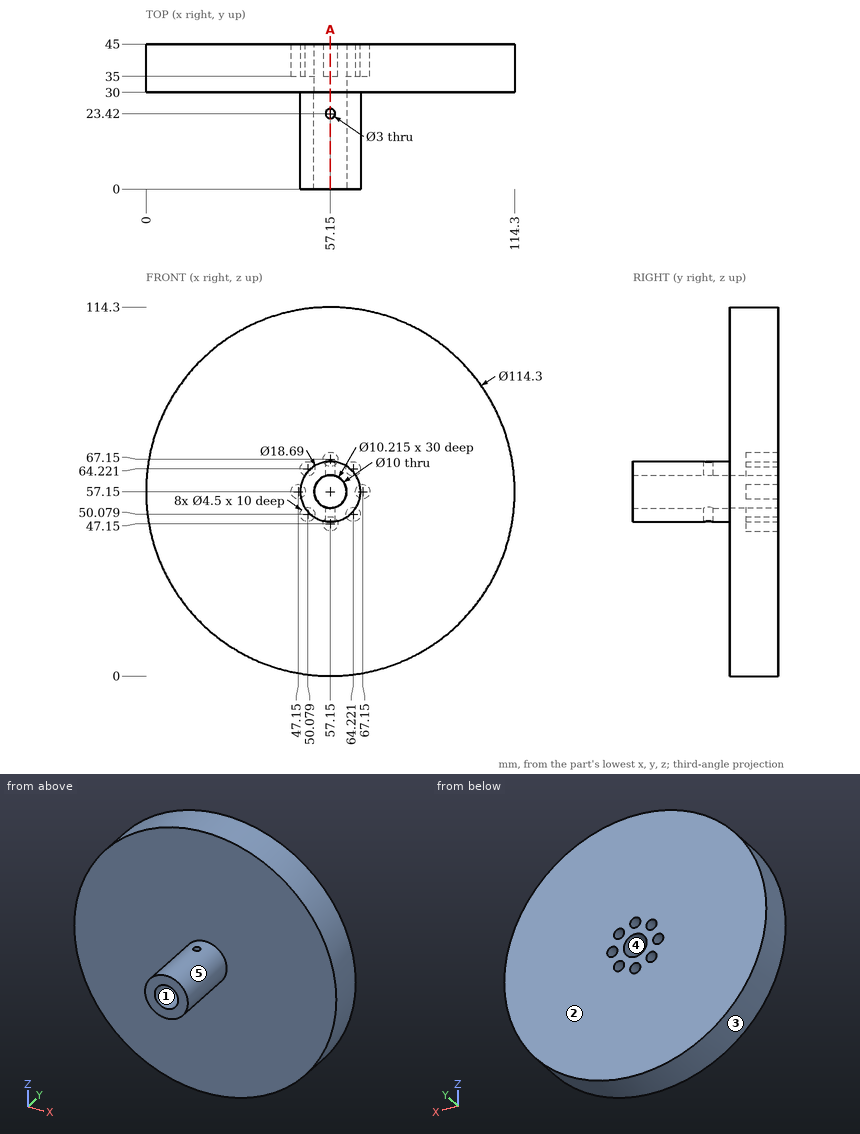
Verification items for this drawing (mm, ordinates from the low corner). A direction names the side the tool comes from. Round coordinates to 2 decimals unless told otherwise and drop trailing zeros. Use one line per item in the form item = value.
1. Go/stop test with flat-tipped pins: pin 1 (2 mm diameter, centred on x = 50.5, z = 51, fed in from +Y); pin 2 (6 mm diameter, centred on x = 84.5, y = 28.5, fed in from -Z); pin 3 (3 mm diameter, centred on y = 39, z = 81, fed in from -X); pin 4 (1.8 mm diameter, centred on x = 57.15, y = 23.42, fed in from +Z). Record where each tip stops, or that it passes through.
Working result:
pin_1 = 35
pin_2 = 5.64
pin_3 = 4.55
pin_4 = through
2. Cross-section at A-A, the plane x = 57.15. Count the separate pieces of the cut face and the enclosed holes in it, plus the area to 3 significant figures.
Working result:
separate_pieces = 4
enclosed_holes = 0
area = 1,700 mm^2
3. Mould release check, pull along X, two halves, no side actions. Record for the marked faces 1, 2 and 3: pulls with the +X half, pulls with the -X half, needs draft (parallel to the pull), parting line crosses it, or undercut.
Working result:
face_1 = undercut
face_2 = needs draft
face_3 = parting line crosses it
4. Set-up check for the marked faces 4 and 5: record each of +Z, -Z, +X, -X, +Y, -Y from which the full face is reachable in a straight line by a thin tool's end or side.
Working result:
face_4 = +Y, -Y
face_5 = -Y
5. Scan lines: line 1 along Z through (x, y) = (57.15, 40.5); line 2 along X through (y, z) = (40, 50); line 3 along Y through (x, z) = (28.5, 73.5). Record each from-to range of solid material in increasing order. Write a range as from..to.
Working result:
line_1 = 0..44.9, 49.4..52.15, 62.15..64.9, 69.4..114.3
line_2 = 0.45..47.83, 52.33..61.97, 66.47..113.85
line_3 = 30..45
